Part model, mm, in its own coordinate system. Face numbers are marked on the shaded views. Round coordinates to 2 decimals unless told otherwise and drop trailing zeros. Order: outer loops, then holes, each group sorted by start corner. A loop starts at its lowest first (then second) coordinate and runs counter-clockwise, first axis right, second up. Notation, with made-up numbers: (-24, 64) -> (13, 64) arc R23 ccw to (13, 87) -> close; hole circle Ø11 at (40, 89). An arc over 180 degrees is marked (long way). Use CSV: the item, a comma, the result in double quotes.
```python
from build123d import *

# Parameters (mm, degrees)
F0_W     = 15.25
F0_H     = 10
F1_DEPTH = 3.8
F2_SIZE2 = 2
F2_SIZE  = 2
F4_DEPTH = 4


with BuildPart() as f1:
    # F0 (on Top) → F1 (new body)
    with BuildSketch(Plane.XY):
        Rectangle(F0_W, F0_H)
    extrude(amount=F1_DEPTH)

    # F2
    f2_edges = [f1.edges().sort_by_distance(p)[0] for p in [
        (0, -5, 3.8),
        (0, 5, 3.8),
    ]]
    chamfer(f2_edges, length=F2_SIZE, length2=F2_SIZE2)

    # F3 (on face) → F4 (cut)
    with BuildSketch(Plane(origin=(0, 0, 0), x_dir=(1, 0, 0), z_dir=(0, 0, -1))):
        Polygon((1.424799, -2.510633), (2.886672, -0.021404), (1.461873, 2.489229), (-1.424799, 2.510633), (-2.886672, 0.021404), (-1.461873, -2.489229), align=None)
    extrude(amount=-F4_DEPTH, mode=Mode.SUBTRACT)


solid = f1.part
```
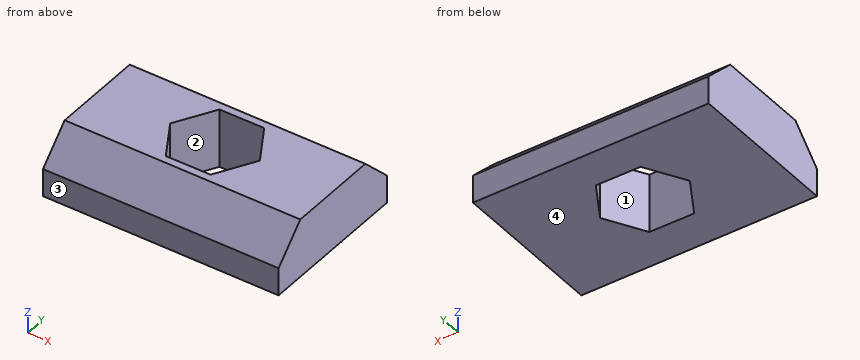
(1) Cut at B-B, the plane y = 0.25. Give the cut face in (x, z) (3 decimals), then the cut area to 3 significant figures.
Reply:
outline,"(-7.625, 0) -> (-2.733, 0) -> (-2.733, 3.8) -> (-7.625, 3.8) -> close; (2.752, 0) -> (7.625, 0) -> (7.625, 3.8) -> (2.752, 3.8) -> close"
area,"37.1 mm2"
(2) Pull direction Y, two halves, no side cores. Call the marked faces 1, 2, 3 and 4: released by +Y, released by -Y, zero draft, split by the parting line, or undercut.
Reply:
face 1,"undercut"
face 2,"undercut"
face 3,"released by -Y"
face 4,"zero draft"
(3) Cut at C-C, the plane x = -1.25. Give the cut face in (y, z), then the cut area to 3 significant figures.
Reply:
outline,"(-5, 0) -> (-2.51, 0) -> (-2.51, 3.8) -> (-3, 3.8) -> (-5, 1.8) -> close; (2.49, 0) -> (5, 0) -> (5, 1.8) -> (3, 3.8) -> (2.49, 3.8) -> close"
area,"15.0 mm2"
(4) Cut at A-A, the plane z = 2.65. Give the cut face in (x, y) (3 decimals).
Reply:
outline,"(-7.625, -4.15) -> (7.625, -4.15) -> (7.625, 4.15) -> (-7.625, 4.15) -> close; hole (-2.887, -0.021) -> (-1.425, -2.511) -> (1.462, -2.489) -> (2.887, 0.021) -> (1.425, 2.511) -> (-1.462, 2.489) -> close"
(5) Cut at D-D, the plane x = 6. Give the cut face in (y, z).
Reply:
outline,"(-5, 0) -> (5, 0) -> (5, 1.8) -> (3, 3.8) -> (-3, 3.8) -> (-5, 1.8) -> close"
(6) Probe probe 1 along Y at (x, z) = (-2, 0.9); probe 2 along X at (y, z) = (0, 1.6) (3 decimals); probe 3 along X at (y, z) = (2, 0.5) (3 decimals). List the from-to ranges inside material, lowest first. Write a range as [from, to].
Reply:
probe 1,"[-5, -1.53], [1.54, 5]"
probe 2,"[-7.625, -2.875], [2.875, 7.625]"
probe 3,"[-7.625, -1.74], [1.725, 7.625]"
